from build123d import *
from OCP.BRepFilletAPI import BRepFilletAPI_MakeChamfer

# Parameters (mm, degrees)
SKETCH1_W           = 43.3
SKETCH1_H           = 24.5
SKETCH1_W_2         = 39.3
SKETCH1_H_2         = 20.5
SKETCH1_H_3         = 12.5
BOSS_EXTRUDE1_DEPTH = 2
SKETCH1_3_W         = 43.3
SKETCH1_3_H         = 24.5
SKETCH1_3_W_2       = 39.3
SKETCH1_3_H_2       = 20.5
BOSS_EXTRUDE2_DEPTH = 15
SKETCH3_W           = 4
SKETCH3_H           = 2
BOSS_EXTRUDE4_DEPTH = 6
CHAMFER2_SIZE       = 3.464101615
CHAMFER2_SIZE_2     = 2
SKETCH4_R           = 0.75
CUT_EXTRUDE1_DEPTH  = 5
SKETCH5_W           = 26.3
SKETCH5_H           = 2
SKETCH5_W_2         = 21.3
CUT_EXTRUDE2_DEPTH  = 13
SKETCH7_W           = 2.5
SKETCH7_H           = 3.5
SKETCH7_H_2         = 3
CUT_EXTRUDE3_DEPTH  = 56.400812268
SKETCH8_W           = 15
SKETCH8_H           = 3.5
SKETCH8_W_2         = 12.5
SKETCH8_H_2         = 3
CUT_EXTRUDE4_DEPTH  = 1
SKETCH9_W           = 3
SKETCH9_H           = 2.5
CUT_EXTRUDE5_DEPTH  = 56.400812268
SKETCH10_W          = 3
SKETCH10_H          = 10
CUT_EXTRUDE6_DEPTH  = 1


with BuildPart() as part:
    # Sketch1 → Boss-Extrude1 (new body)
    # profile 1 of 4: a face of its own
    with BuildSketch(Plane(origin=(0, 0, 0), x_dir=(1, 0, 0), z_dir=(0, 1, 0))):
        with Locations((19.45, 10.05)):
            Rectangle(SKETCH1_W, SKETCH1_H)
        with Locations((19.45, 10.05)):
            Rectangle(SKETCH1_W_2, SKETCH1_H_2, mode=Mode.SUBTRACT)
    # profile 2 of 4: a face of its own
    with BuildSketch(Plane(origin=(0, 0, 0), x_dir=(1, 0, 0), z_dir=(0, 1, 0))):
        with Locations((19.45, 10.05)):
            Rectangle(SKETCH1_W_2, SKETCH1_H_2)
    # profile 3 of 4: a face of its own
    with BuildSketch(Plane(origin=(0, 0, 0), x_dir=(1, 0, 0), z_dir=(0, 1, 0))):
        with Locations((19.45, -8.45)):
            Rectangle(SKETCH1_W, SKETCH1_H_3)
    # profile 4 of 4: a face of its own
    with BuildSketch(Plane(origin=(0, 0, 0), x_dir=(1, 0, 0), z_dir=(0, 1, 0))):
        with Locations((19.45, 28.55)):
            Rectangle(SKETCH1_W, SKETCH1_H_3)
    extrude(amount=BOSS_EXTRUDE1_DEPTH)

    # Sketch1<3> → Boss-Extrude2 (add)
    with BuildSketch(Plane(origin=(0, 0, 0), x_dir=(1, 0, 0), z_dir=(0, 1, 0))):
        with Locations((19.45, 10.05)):
            Rectangle(SKETCH1_3_W, SKETCH1_3_H)
        with Locations((19.45, 10.05)):
            Rectangle(SKETCH1_3_W_2, SKETCH1_3_H_2, mode=Mode.SUBTRACT)
    extrude(amount=BOSS_EXTRUDE2_DEPTH)

    # Sketch3 → Boss-Extrude4 (add)
    with BuildSketch(Plane(origin=(0, 15, 0), x_dir=(1, 0, 0), z_dir=(0, 1, 0))):
        with Locations((-0.2, -3.2)):
            Rectangle(SKETCH3_W, SKETCH3_H)
        with Locations((39.1, -3.2)):
            Rectangle(SKETCH3_W, SKETCH3_H)
        with Locations((39.1, 23.3)):
            Rectangle(SKETCH3_W, SKETCH3_H)
        with Locations((-0.2, 23.3)):
            Rectangle(SKETCH3_W, SKETCH3_H)
    extrude(amount=-BOSS_EXTRUDE4_DEPTH)

    # Chamfer2
    chamfer2_edges_1 = [part.edges().sort_by_distance(p)[0] for p in [
        (-0.2, 9, -22.3),
    ]]
    chamfer2_side_1 = [part.faces().sort_by_distance(p)[0] for p in [
        (-0.2, 8.96, -22.3),
    ]]
    chamfer2_edges_2 = [part.edges().sort_by_distance(p)[0] for p in [
        (39.1, 9, -22.3),
    ]]
    chamfer2_side_2 = [part.faces().sort_by_distance(p)[0] for p in [
        (39.1, 9, -22.34),
    ]]
    chamfer2_edges_3 = [part.edges().sort_by_distance(p)[0] for p in [
        (39.1, 9, 2.2),
    ]]
    chamfer2_side_3 = [part.faces().sort_by_distance(p)[0] for p in [
        (39.1, 9, 2.24),
    ]]
    chamfer2_edges_4 = [part.edges().sort_by_distance(p)[0] for p in [
        (-0.2, 9, 2.2),
    ]]
    chamfer2_side_4 = [part.faces().sort_by_distance(p)[0] for p in [
        (-0.2, 9, 2.24),
    ]]
    chamfer2 = BRepFilletAPI_MakeChamfer(part.part.solid().wrapped)
    for e in chamfer2_edges_1:
        chamfer2.Add(CHAMFER2_SIZE - 0.0001, CHAMFER2_SIZE_2 - 0.0001, e.wrapped, chamfer2_side_1[0].wrapped)
    for e in chamfer2_edges_2:
        chamfer2.Add(CHAMFER2_SIZE_2 - 0.0001, CHAMFER2_SIZE - 0.0001, e.wrapped, chamfer2_side_2[0].wrapped)
    for e in chamfer2_edges_3:
        chamfer2.Add(CHAMFER2_SIZE_2 - 0.0001, CHAMFER2_SIZE - 0.0001, e.wrapped, chamfer2_side_3[0].wrapped)
    for e in chamfer2_edges_4:
        chamfer2.Add(CHAMFER2_SIZE_2 - 0.0001, CHAMFER2_SIZE - 0.0001, e.wrapped, chamfer2_side_4[0].wrapped)
    add(Compound.cast(chamfer2.Shape()), mode=Mode.REPLACE)  # a hair under: the kernel refuses the full size

    # Sketch4 → Cut-Extrude1 (cut)
    with BuildSketch(Plane(origin=(0, 15, 0), x_dir=(1, 0, 0), z_dir=(0, 1, 0))):
        with Locations(Location((-0.2, 22.3, 0), (0, 0, 270))):
            Circle(SKETCH4_R)
        with Locations(Location((-0.2, -2.2, 0), (0, 0, 270))):
            Circle(SKETCH4_R)
        with Locations(Location((39.1, -2.2, 0), (0, 0, 270))):
            Circle(SKETCH4_R)
        with Locations(Location((39.1, 22.3, 0), (0, 0, 270))):
            Circle(SKETCH4_R)
    extrude(amount=-CUT_EXTRUDE1_DEPTH, mode=Mode.SUBTRACT)

    # Sketch5 → Cut-Extrude2 (cut)
    with BuildSketch(Plane(origin=(0, 15, 0), x_dir=(1, 0, 0), z_dir=(0, 1, 0))):
        with Locations((21.95, 21.3)):
            Rectangle(SKETCH5_W, SKETCH5_H)
        with Locations((19.45, -1.2)):
            Rectangle(SKETCH5_W_2, SKETCH5_H)
    extrude(amount=-CUT_EXTRUDE2_DEPTH, mode=Mode.SUBTRACT)

    # Sketch7 → Cut-Extrude3 (cut, through all)
    with BuildSketch(Plane(origin=(0, 2, 0), x_dir=(1, 0, 0), z_dir=(0, 1, 0))):
        with Locations((16.35, 32.05)):
            Rectangle(SKETCH7_W, SKETCH7_H)
        with Locations((33.85, 32.05)):
            Rectangle(SKETCH7_W, SKETCH7_H)
        with Locations((13.35, -11.7)):
            Rectangle(SKETCH7_W, SKETCH7_H_2)
        with Locations((28.35, -11.7)):
            Rectangle(SKETCH7_W, SKETCH7_H_2)
    extrude(amount=-CUT_EXTRUDE3_DEPTH, mode=Mode.SUBTRACT)

    # Sketch8 → Cut-Extrude4 (cut)
    with BuildSketch(Plane.XZ):
        with Locations((25.1, -32.05)):
            Rectangle(SKETCH8_W, SKETCH8_H)
        with Locations((20.85, 11.7)):
            Rectangle(SKETCH8_W_2, SKETCH8_H_2)
    extrude(amount=-CUT_EXTRUDE4_DEPTH, mode=Mode.SUBTRACT)

    # Sketch9 → Cut-Extrude5 (cut, through all)
    with BuildSketch(Plane(origin=(0, 2, 0), x_dir=(1, 0, 0), z_dir=(0, 1, 0))):
        with Locations((0.3, 23.55)):
            Rectangle(SKETCH9_W, SKETCH9_H)
    extrude(amount=-CUT_EXTRUDE5_DEPTH, mode=Mode.SUBTRACT)

    # Sketch10 → Cut-Extrude6 (cut)
    with BuildSketch(Plane.XZ):
        with Locations((0.3, -29.8)):
            Rectangle(SKETCH10_W, SKETCH10_H)
    extrude(amount=-CUT_EXTRUDE6_DEPTH, mode=Mode.SUBTRACT)


solid = part.part
The model under review builds one solid part; all positions refer to its coordinate system, in mm. A direction names the side the tool comes from. Round coordinates to 2 decimals unless told otherwise and drop trailing zeros. Order: outer loops, then holes, each group sorted by start corner. A loop starts at its lowest first (then second) coordinate and runs counter-clockwise, first axis right, second up. Notation, with made-up numbers: (81, 88) -> (108, 88) arc R30 ccw to (108, 116) -> close; hole circle Ø2 at (-12.5, 71.25). An arc over 180 degrees is marked (long way). Return JSON: item names as keys, results as strings.
1. For faces 1 (the face through (12.1, 1, 12)), 2 (the face through (0, 10, -22)), 3 (the face through (34, 8, 2.2)), 4 (the face through (0, 1, -30)), 5 (the face through (-0.228, 7.292, -23.314)), list the 3-axis set-ups (+Z, -Z, +X, -X, +Y, -Y) from which the entire face can be reached by the end or side of a thin tool; tool diameter is ignored.
Answer block:
{"face 1": "+Y, -Y", "face 2": "+Y", "face 3": "+Z", "face 4": "-Z, -Y", "face 5": "-Z, +X, -X"}
2. The part is to be moulded in two halves that separate along Z. For faces 6 (the face through (0, 12, 4.2)), 7 (the face through (21, 1, 12)), 8 (the face through (36.7, 7, -22.3)), 9 (the face through (37.1, 11, -23)), say which applies: +Z half, -Z half, draft (parallel to the pull), parting line (faces both ways), or undercut.
Answer block:
{"face 6": "+Z half", "face 7": "undercut", "face 8": "-Z half", "face 9": "draft"}
3. Take a section at B-B (x = 16.5). Write out the cut boundary in (y, z).
Answer block:
{"outline": "(0, -34.8) -> (2, -34.8) -> (2, -33.8) -> (0, -33.8) -> close; (0, -30.3) -> (2, -30.3) -> (2, 14.7) -> (0, 14.7) -> (0, 13.2) -> (1, 13.2) -> (1, 10.2) -> (0, 10.2) -> close"}
4. Take a section at D-D (z = -18.5). Write out the cut boundary in (x, y).
Answer block:
{"outline": "(-2.2, 0) -> (41.1, 0) -> (41.1, 15) -> (39.1, 15) -> (39.1, 2) -> (-0.2, 2) -> (-0.2, 15) -> (-2.2, 15) -> close"}
5. Take a section at A-A (y = 13.5). Write out the cut boundary in (x, z).
Answer block:
{"outline": "(-2.2, -24.3) -> (1.8, -24.3) -> (1.8, -22.3) -> (8.8, -22.3) -> (8.8, -20.3) -> (-0.2, -20.3) -> (-0.2, 0.2) -> (8.8, 0.2) -> (8.8, 2.2) -> (1.8, 2.2) -> (1.8, 4.2) -> (-2.2, 4.2) -> close; (30.1, 0.2) -> (39.1, 0.2) -> (39.1, -20.3) -> (35.1, -20.3) -> (35.1, -22.3) -> (37.1, -22.3) -> (37.1, -24.3) -> (41.1, -24.3) -> (41.1, 4.2) -> (37.1, 4.2) -> (37.1, 2.2) -> (30.1, 2.2) -> close; hole circle Ø1.5 at (-0.2, -22.3); hole circle Ø1.5 at (-0.2, 2.2); hole circle Ø1.5 at (39.1, -22.3); hole circle Ø1.5 at (39.1, 2.2)"}
6. For L1, parallel to Z at x = 5, y = 8.75; L2, parallel to X at y = 5, z = -9; L3, parallel to Z at x = 35, y = 12.5, list the stretches that pass through material, from the lowest coordinate up. Write a range as [from, to].
Answer block:
{"L1": "z = [-22.3, -20.3], [0.2, 2.2]", "L2": "x = [-2.2, -0.2], [39.1, 41.1]", "L3": "z = [0.2, 2.2]"}
7. Insertion check: P1, Ø3, axis at x = 7.5, y = 10, coming from the -Z side; P2, Ø9, axis at x = 6, y = 9, coming from the +Z side; P3, Ø5, axis at x = 37.5, y = 10.5, coming from the -Z side. Each pin has a flat end and moves straight along its axis. Give the tip position at first contact, or say it passes through.
Answer block:
{"P1": "stops at z = -22.3", "P2": "stops at z = 4.2", "P3": "stops at z = -24.3"}
8. Take a section at C-C (y = 3.75). Write out the cut boundary in (x, z).
Answer block:
{"outline": "(-2.2, -22.3) -> (8.8, -22.3) -> (8.8, -20.3) -> (-0.2, -20.3) -> (-0.2, 0.2) -> (8.8, 0.2) -> (8.8, 2.2) -> (-2.2, 2.2) -> close; (30.1, 0.2) -> (39.1, 0.2) -> (39.1, -20.3) -> (35.1, -20.3) -> (35.1, -22.3) -> (41.1, -22.3) -> (41.1, 2.2) -> (30.1, 2.2) -> close"}
